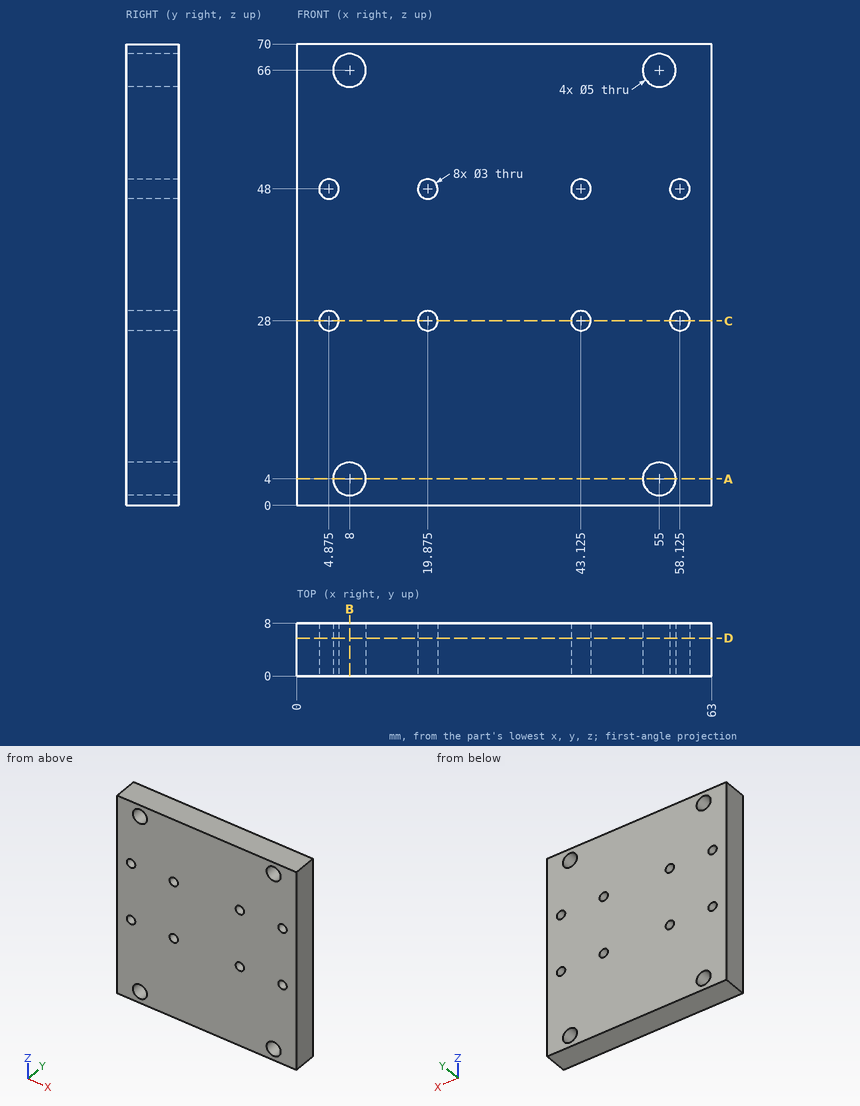
Verification items for this drawing (mm, ordinates from the low corner). Coordinates: 2 decimals unless noted, no trailing zeros. Write each loop counter-clockwise with the first axis right and the second up, starting at its lowest first coordinate (ties: lowest second). Pieces come first, ordered by that corner, then holes. Notation, with made-up numbers: M 33.25,-2 L 75.25,-2 A11 cw 75.25,10 Z; hole C 0,37 d2. An arc over 180 degrees is marked long. Answer as a JSON object with one key per item and string values. Group by question number.
(1) Cross-section at B-B, the plane x = 8. Record the cut outline in (y, z).
(2) Cross-section at C-C, the plane z = 28. Record the cut outline in (x, y) (3 decimals), and give its area (3 significant figures).
(3) Cross-section at A-A, the plane z = 4. Record the cut outline in (x, y), and give its area (3 significant figures).
(4) Cross-section at D-D, the plane y = 5.75. State how many separate pieces and enclosed holes the cut face has, and give its area (3 significant figures).
(5) Material ranges on line 1 (X direction, y = 1.75, z = 66); line 2 (Z direction, x = 55, y = 5); line 3 (X direction, y = 6.25, z = 28) (3 decimals), recorded low to high.
(6) Gauge pin test, flat end, axial feed: pin 1 (8 mm diameter, centred on x = 55, z = 4, fed in from -Y). Record the tip position at first contact, or that the pin passes through.
Reply:
{
 "1": {"outline": "M 0,0 L 8,0 L 8,1.5 L 0,1.5 Z; M 0,6.5 L 8,6.5 L 8,63.5 L 0,63.5 Z; M 0,68.5 L 8,68.5 L 8,70 L 0,70 Z"},
 "2": {"outline": "M 0,0 L 3.375,0 L 3.375,8 L 0,8 Z; M 6.375,0 L 18.375,0 L 18.375,8 L 6.375,8 Z; M 21.375,0 L 41.625,0 L 41.625,8 L 21.375,8 Z; M 44.625,0 L 56.625,0 L 56.625,8 L 44.625,8 Z; M 59.625,0 L 63,0 L 63,8 L 59.625,8 Z", "area": "408 mm²"},
 "3": {"outline": "M 0,0 L 5.5,0 L 5.5,8 L 0,8 Z; M 10.5,0 L 52.5,0 L 52.5,8 L 10.5,8 Z; M 57.5,0 L 63,0 L 63,8 L 57.5,8 Z", "area": "424 mm²"},
 "4": {"separate pieces": "1", "enclosed holes": "12", "area": "4,270 mm²"},
 "5": {"line 1": "0 to 5.5, 10.5 to 52.5, 57.5 to 63", "line 2": "0 to 1.5, 6.5 to 63.5, 68.5 to 70", "line 3": "0 to 3.375, 6.375 to 18.375, 21.375 to 41.625, 44.625 to 56.625, 59.625 to 63"},
 "6": {"pin 1": "y = 0"}
}
